from build123d import *

# Parameters (mm, degrees)
SKETCH1_W           = 66
SKETCH1_H           = 42
SKETCH1_R           = 1
SKETCH1_W_2         = 15
SKETCH1_H_2         = 7
BOSS_EXTRUDE1_DEPTH = 1


with BuildPart() as part:
    # Sketch1 → Boss-Extrude1 (new body)
    with BuildSketch(Plane(origin=(0, 0, 0), x_dir=(1, 0, 0), z_dir=(0, 1, 0))):
        Rectangle(SKETCH1_W, SKETCH1_H)
        with Locations((-30, -18)):
            Circle(SKETCH1_R, mode=Mode.SUBTRACT)
        with Locations((30, -18)):
            Circle(SKETCH1_R, mode=Mode.SUBTRACT)
        with Locations((30, 18)):
            Circle(SKETCH1_R, mode=Mode.SUBTRACT)
        with Locations((-30, 18)):
            Circle(SKETCH1_R, mode=Mode.SUBTRACT)
        with Locations((-17.5, -12.5)):
            Rectangle(SKETCH1_W_2, SKETCH1_H_2, mode=Mode.SUBTRACT)
        with Locations((17.5, -12.5)):
            Rectangle(SKETCH1_W_2, SKETCH1_H_2, mode=Mode.SUBTRACT)
        with Locations((17.5, 12.5)):
            Rectangle(SKETCH1_W_2, SKETCH1_H_2, mode=Mode.SUBTRACT)
        with Locations((-17.5, 12.5)):
            Rectangle(SKETCH1_W_2, SKETCH1_H_2, mode=Mode.SUBTRACT)
    extrude(amount=BOSS_EXTRUDE1_DEPTH)


solid = part.part
Verification items for the finished model (mm, model axes). Round coordinates to 2 decimals unless told otherwise and drop trailing zeros. Order: outer loops, then holes, each group sorted by start corner. A loop starts at its lowest first (then second) coordinate and runs counter-clockwise, first axis right, second up.
1. Section check A-A on x = 22. Record the cut outline in (y, z).
Final values:
outline: (0, -21) - (1, -21) - (1, -16) - (0, -16) - close; (0, -9) - (1, -9) - (1, 9) - (0, 9) - close; (0, 16) - (1, 16) - (1, 21) - (0, 21) - close
2. Release check for a two-part mould opening along Z. For faces 1 (the flat face through (0, 0, 0)), 2 (the cylindrical face through (29.783, 0.493, -17.024)) record: +Z half, -Z half, draft (parallel to the pull), parting line (faces both ways), or undercut.
Final values:
face 1: draft
face 2: undercut
3. Section check C-C on z = 18. Record the cut outline in (x, y).
Final values:
outline: (-33, 0) - (-31, 0) - (-31, 1) - (-33, 1) - close; (-29, 0) - (29, 0) - (29, 1) - (-29, 1) - close; (31, 0) - (33, 0) - (33, 1) - (31, 1) - close
4. Section check B-B on y = 0.35. State how many separate pieces and enclosed holes the cut face has, then the cut area to 3 significant figures.
Final values:
separate pieces: 1
enclosed holes: 8
area: 2,340 mm2
5. Thickness scan on L1, parallel to Z at x = 20, y = 0.75; L2, parallel to X at y = 0.7, z = 18; L3, parallel to Z at x = 30, y = 0.75. Record the ranges inside material, lowest first.
Final values:
L1: z = -21 to -16, -9 to 9, 16 to 21
L2: x = -33 to -31, -29 to 29, 31 to 33
L3: z = -21 to -19, -17 to 17, 19 to 21
6. Go/stop test with a flat-tipped pin: P1, Ø4, axis at x = 9, z = 13.5, coming from the -Y side. Record where the tip stops, or that it passes through.
Final values:
P1: stops at y = 0
